Here's how the part is built. I have some questions about the finished solid (model axes, mm). Coordinates: 2 decimals unless noted, no trailing zeros. Write each loop counter-clockwise with the first axis right and the second up, starting at its lowest first coordinate (ties: lowest second). Pieces come first, ordered by that corner, then holes. Notation, with made-up numbers: (-28, 44.5) -> (31, 44.5) arc R29 ccw to (31, 81.5) -> close; hole circle Ø1 at (27, -31). An arc over 180 degrees is marked (long way). Use a Markdown table: item, result. Add a question column.
Autodesk Inventor part; units mm, degrees
ref_plane "FDT_KSAUFSATZ_XY" through (0, 0, 26) normal (0, 0, 1) x (-1, 0, 0)
ref_plane "FDT_KSAUFSATZ_YZ" through (0, 0, 26) normal (-1, 0, 0) x (0, -1, 0)
ref_plane "FDT_KSAUFSATZ_ZX" through (0, 0, 26) normal (0, -1, 0) x (0, 0, 1)
sketch "Sketch_2" plane through (0, 0, 0) normal (1, 0, 0) x (0, 1, 0)
  line L0 (0, -588.95) -> (0, 12)
  line L1 (0, 12) -> (10, 12)
  line L2 (10, 12) -> (10, -573.2)
  line L3 (10, -573.2) -> (31.5, -573.2)
  line L4 (31.5, -573.2) -> (31.5, -588.95)
  line L5 (31.5, -588.95) -> (0, -588.95)
  line L6 (0, -588.95) -> (0, 12)
revolve "Revolution1" add sketch "Sketch_2" angle 360 about axis through (0, 0, -588.95) along (0, 0, -1)
sketch "Sketch_6" plane through (0, 0, 0) normal (1, 0, 0) x (0, 1, 0)
  line L0 (0, 11) -> (0, 44)
  line L1 (0, 44) -> (7.08, 44)
  line L2 (7.08, 44) -> (8, 43.08)
  line L3 (8, 43.08) -> (8, 17.4849)
  line L4 (8, 17.4849) -> (6.9952, 14.7243)
  arc A0 (6.9952, 14.7243) -> (6.95, 14.4678) centre (7.7, 14.4678) ccw
  line L5 (6.95, 14.4678) -> (6.95, 12.75)
  arc A1 (6.95, 12.75) -> (7.7, 12) centre (7.7, 12.75) ccw
  line L6 (7.7, 12) -> (8, 12)
  line L7 (8, 12) -> (8, 11)
  line L8 (8, 11) -> (0, 11)
  line L9 (0, 11) -> (0, 44)
revolve "Revolution2" add sketch "Sketch_6" angle 360 about axis through (0, 0, 11) along (0, 0, -1)
thread "Thread1"
sketch "Sketch_7" plane through (0, 0, 4) normal (0, 0, 1) x (1, 0, 0)
  line L0 (-17, 34) -> (-17, -17)
  line L1 (-17, -17) -> (-8.5, -17)
  line L2 (-8.5, -17) -> (-8.5, 17)
  line L3 (-8.5, 17) -> (8.5, 17)
  line L4 (8.5, 17) -> (8.5, -17)
  line L5 (8.5, -17) -> (17, -17)
  line L6 (17, -17) -> (17, 34)
  line L7 (17, 34) -> (-17, 34)
extrude "Extrusion1" cut sketch "Sketch_7" along normal blind 9
ref_plane "FDT_KSAUFSATZ_XY" through (0, 0, 26) normal (0, 0, 1) x (-1, 0, 0)
ref_plane "FDT_KSAUFSATZ_YZ" through (0, 0, 26) normal (-1, 0, 0) x (0, -1, 0)
ref_plane "FDT_KSAUFSATZ_ZX" through (0, 0, 26) normal (0, -1, 0) x (0, 0, 1)
ref_plane "FDT_NUT_XY" through (0, 0, 26) normal (0, 0, 1) x (-1, 0, 0)
ref_plane "FDT_NUT_YZ" through (0, 0, 26) normal (-1, 0, 0) x (0, -1, 0)
ref_plane "FDT_NUT_ZX" through (0, 0, 26) normal (0, -1, 0) x (0, 0, 1)
ref_plane "KS_XY" through (0, 0, 0) normal (0, 0, -1) x (1, 0, 0)
ref_plane "KS_YZ" through (0, 0, 0) normal (1, 0, 0) x (0, -1, 0)
ref_plane "KS_ZX" through (0, 0, 0) normal (0, -1, 0) x (0, 0, -1)
ref_plane "NUT1_XY" through (0, 0, 32) normal (0, 0, 1) x (1, 0, 0)
ref_plane "NUT1_YZ" through (0, 0, 32) normal (1, 0, 0) x (0, 1, 0)
ref_plane "NUT1_ZX" through (0, 0, 32) normal (0, 1, 0) x (0, 0, 1)
properties part number "193995 DSNU-63-500-P---(A---00--0-KS)" material "Aluminum 6061"
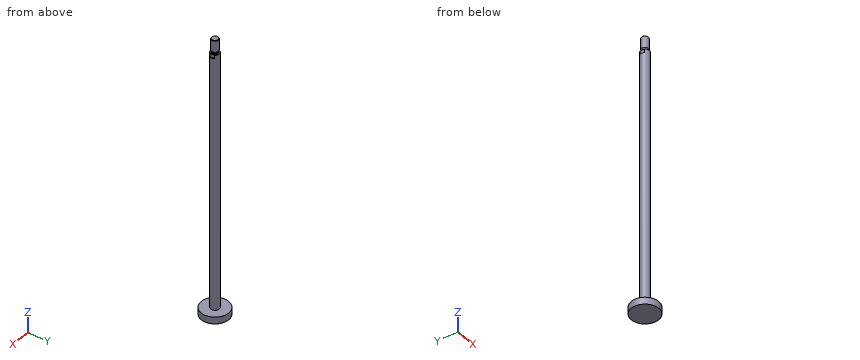
Q1. Suppose I cut it at B-B, the plane y = 0. Write out the boundary of the cut face in (x, z), and give its area (3 significant figures).
Q2. Suppose I cut it at C-C, the plane z = -367.5. Write out the boundary of the cut face in (x, y), and give its area (3 significant figures).
Q3. Suppose I cut it at A-A, the plane x = 0. Write out the boundary of the cut face in (y, z).
Q4. Will these pins go through, and if not, where does the flat tip stop? pin 1 (3 mm diameter, centred on x = -8.5, z = -310.5, fed in from +Y); pin 2 (2.5 mm diameter, centred on y = 0, z = 7, fed in from -X); pin 3 (1.2 mm diameter, centred on x = 9, y = -1, fed in from +Z); pin 4 (6 mm diameter, centred on y = 14.5, z = -207.5, fed in from -X).
Q5. Please list where these lines run through material, in increasing order: line 1 (Y direction, x = -1.5, z = -285); line 2 (Z direction, x = 22, y = 19.5); line 3 (Z direction, x = 4.5, y = 6).
Answer key:
| question | item | result |
|---|---|---|
| 1 | outline | (-31.5, -588.95) -> (31.5, -588.95) -> (31.5, -573.2) -> (10, -573.2) -> (10, 4) -> (8.5, 4) -> (8.5, 12) -> (7.7, 12) arc R0.75 cw to (6.95, 12.75) -> (6.95, 14.47) arc R0.75 cw to (7, 14.72) -> (8, 17.48) -> (8, 43.08) -> (7.08, 44) -> (-7.08, 44) -> (-8, 43.08) -> (-8, 17.48) -> (-7, 14.72) arc R0.75 cw to (-6.95, 14.47) -> (-6.95, 12.75) arc R0.75 cw to (-7.7, 12) -> (-8.5, 12) -> (-8.5, 4) -> (-10, 4) -> (-10, -573.2) -> (-31.5, -573.2) -> close |
| 1 | area | 13,200 mm^2 |
| 2 | outline | circle Ø20 at (0, 0) |
| 2 | area | 314 mm^2 |
| 3 | outline | (-31.5, -588.95) -> (31.5, -588.95) -> (31.5, -573.2) -> (10, -573.2) -> (10, 12) -> (7.7, 12) arc R0.75 cw to (6.95, 12.75) -> (6.95, 14.47) arc R0.75 cw to (7, 14.72) -> (8, 17.48) -> (8, 43.08) -> (7.08, 44) -> (-7.08, 44) -> (-8, 43.08) -> (-8, 17.48) -> (-7, 14.72) arc R0.75 cw to (-6.95, 14.47) -> (-6.95, 12.75) arc R0.75 cw to (-7.7, 12) -> (-10, 12) -> (-10, -573.2) -> (-31.5, -573.2) -> close |
| 4 | pin 1 | stops at y = 7.14 |
| 4 | pin 2 | stops at x = -8.5 |
| 4 | pin 3 | stops at z = 12 |
| 4 | pin 4 | passes through |
| 5 | line 1 | y = -9.89 to 9.89 |
| 5 | line 2 | z = -588.95 to -573.2 |
| 5 | line 3 | z = -588.95 to 12.03, 16.11 to 43.58 |
